Verification items for the finished model (mm, model axes). Coordinates: 2 decimals unless noted, no trailing zeros. Loops run counter-clockwise (first coordinate to the right, second up) from the corner with the lowest first, then second, coordinate; pieces in that order, holes last. Notation, with made-up numbers: (-21, -18.75) -> (37, -18.75) arc R24 ccw to (37, -7.75) -> close; hole circle Ø10 at (36, 41). An arc over 180 degrees is marked (long way). Answer as a JSON object with one key per item and string values. Group by question number.
Q1. Gauge pin test, flat end, axial feed: pin 1 Ø1.5 at (y, z) = (3.5, -2.5) entering from +X. Record the tip position at first contact, or that the pin passes through.
Q2. Cross-section at A-A on y = 5. Record the boundary of the cut face in (x, z) (1 decimal), and give its area (3 significant figures).
Q3. Scan lines: L1, parallel to Z at x = -1.75, y = 5.5; L2, parallel to Z at x = 0.5, y = 8.25; L3, parallel to X at y = 4.75, z = 0.75. Record each from-to range of solid material in increasing order.
```python
from build123d import *

# Parameters (mm, degrees)
SKETCH1_R           = 4.7625
BOSS_EXTRUDE1_DEPTH = 9.525
SKETCH2_OUTSIDE_W   = 60.842
SKETCH2_OUTSIDE_H   = 58.14
SKETCH2_OUTSIDE_R   = 8.7376
CUT_EXTRUDE1_DEPTH  = 9.525
CUT_EXTRUDE1_TAPER  = 60
SKETCH3_OUTSIDE_W   = 60.842
SKETCH3_OUTSIDE_H   = 58.14
SKETCH3_OUTSIDE_R   = 8.7376
CUT_EXTRUDE2_DEPTH  = 9.525
CUT_EXTRUDE2_TAPER  = 60
CHAMFER1_SIZE       = 0.635


with BuildPart() as part:
    # Sketch1 → Boss-Extrude1 (new body)
    with BuildSketch(Plane(origin=(0, 0, 0), x_dir=(1, 0, 0), z_dir=(0, 1, 0))):
        Polygon((10.089311424, 0), (5.044655712, 8.7376), (-5.044655712, 8.7376), (-10.089311424, 0), (-5.044655712, -8.7376), (5.044655712, -8.7376), align=None)
        Circle(SKETCH1_R, mode=Mode.SUBTRACT)
    extrude(amount=BOSS_EXTRUDE1_DEPTH)

    # Sketch2 outside → Cut-Extrude1 (cut)
    with BuildSketch(Plane(origin=(0, 9.525, 0), x_dir=(1, 0, 0), z_dir=(0, 1, 0))):
        Rectangle(SKETCH2_OUTSIDE_W, SKETCH2_OUTSIDE_H)
        Circle(SKETCH2_OUTSIDE_R, mode=Mode.SUBTRACT)
    extrude(amount=-CUT_EXTRUDE1_DEPTH, taper=CUT_EXTRUDE1_TAPER, mode=Mode.SUBTRACT)

    # Sketch3 outside → Cut-Extrude2 (cut)
    with BuildSketch(Plane.XZ):
        Rectangle(SKETCH3_OUTSIDE_W, SKETCH3_OUTSIDE_H)
        Circle(SKETCH3_OUTSIDE_R, mode=Mode.SUBTRACT)
    extrude(amount=-CUT_EXTRUDE2_DEPTH, taper=CUT_EXTRUDE2_TAPER, mode=Mode.SUBTRACT)

    # Chamfer1
    chamfer1_edges = [part.edges().sort_by_distance(p)[0] for p in [
        (-4.7625, 0, 0),
        (-4.7625, 9.525, 0),
    ]]
    chamfer(chamfer1_edges, length=CHAMFER1_SIZE)


solid = part.part
```
Computed values:
{
 "1": {"pin 1": "stops at x = 9.08"},
 "2": {"outline": "(-10.1, 0) -> (-5, -8.7) -> (5, -8.7) -> (10.1, 0) -> (5, 8.7) -> (-5, 8.7) -> close; hole circle Ø9.5 at (0, 0)", "area": "193 mm²"},
 "3": {"L1": "z = -8.74 to -4.43, 4.43 to 8.74", "L2": "z = -8.74 to -4.74, 4.74 to 8.74", "L3": "x = -9.66 to -4.7, 4.7 to 9.66"}
}
